Geometry check sheet. Reference: the model listing, model coordinates, mm. A direction names the side the tool comes from. Round coordinates to 2 decimals unless told otherwise and drop trailing zeros. Loops run counter-clockwise (first coordinate to the right, second up) from the corner with the lowest first, then second, coordinate; pieces in that order, holes last. Notation, with made-up numbers: (72.25, 40.5) - (112.25, 40.5) arc R15 cw to (112.25, 62.5) - close; hole circle Ø9 at (75.5, 75.5). An arc over 180 degrees is marked (long way). Write item = value, one per line.
```python
from build123d import *

# Parameters (mm, degrees)
EXTRUDE_1_DEPTH = 1.5
EXTRUDE_2_DEPTH = 1
FILLET_1_R      = 0.5


with BuildPart() as part:
    # 草图1 → 凸台-拉伸1 (new body)
    with BuildSketch(Plane(origin=(0, 0, 0), x_dir=(1, 0, 0), z_dir=(0, 1, 0))):
        Polygon((-24.5, 13), (24.5, 13), (24.5, -13), (7.05, -13), (7.05, -26), (7.05, -27.5), (-7.05, -27.5), (-7.05, -26), (-7.05, -13), (-24.5, -13), align=None)
    extrude(amount=EXTRUDE_1_DEPTH)

    # 草图2 → 凸台-拉伸2 (add)
    with BuildSketch(Plane(origin=(0, 1.5, 0), x_dir=(1, 0, 0), z_dir=(0, 1, 0))):
        Polygon((23, 11.5), (23, -11.5), (5.55, -11.5), (5.55, -13), (5.55, -24.5), (5.55, -26), (-5.55, -26), (-5.55, -24.5), (-5.55, -13), (-5.55, -11.5), (-23, -11.5), (-23, 11.5), align=None)
    extrude(amount=EXTRUDE_2_DEPTH)

    # 圆角1
    fillet_1_edges = [part.edges().sort_by_distance(p)[0] for p in [
        (7.05, 0, 20.25),
        (0, 0, 27.5),
        (-7.05, 0, 20.25),
        (-15.775, 0, 13),
        (-24.5, 0, 0),
        (0, 0, -13),
        (24.5, 0, 0),
        (15.775, 0, 13),
    ]]
    fillet(fillet_1_edges, radius=FILLET_1_R)


solid = part.part
```
(1) Gauge pin test, flat ends, axial feed: pin 1 (0.5 mm diameter, centred on y = 1, z = 22.5, fed in from +X); pin 2 (0.5 mm diameter, centred on y = 2, z = -1, fed in from -X); pin 3 (0.8 mm diameter, centred on x = -4.5, y = 2, fed in from -Z). Record the tip position at first contact, or that the pin passes through.
Answers follow:
pin_1 = 7.05
pin_2 = -23
pin_3 = -11.5
(2) Section check C-C (z = 24). Enter the section's corners in (x, y), then the cut area to 3 significant figures.
Answers follow:
outline = (-7.05, 0.5) arc R0.5 ccw to (-6.55, 0) - (6.55, 0) arc R0.5 ccw to (7.05, 0.5) - (7.05, 1.5) - (5.55, 1.5) - (5.55, 2.5) - (-5.55, 2.5) - (-5.55, 1.5) - (-7.05, 1.5) - close
area = 32.1 mm²
(3) Set-up check for faces 1 (the flat face through (16, 1, 13)), 2 (the flat face through (-14, 2, 11.5)), 3 (the flat face through (-23, 2, 0)), 4 (the flat face through (23, 2, 0)): record each of +Z, -Z, +X, -X, +Y, -Y from which the full face is reachable in a straight line by a thin tool's end or side.
Answers follow:
face_1 = +Z, +X, +Y, -Y
face_2 = +Z, -X, +Y
face_3 = +Z, -Z, -X, +Y
face_4 = +Z, -Z, +X, +Y
(4) Section check A-A (y = 1.9). Enter the section's corners in (x, z).
Answers follow:
outline = (-23, -11.5) - (23, -11.5) - (23, 11.5) - (5.55, 11.5) - (5.55, 26) - (-5.55, 26) - (-5.55, 11.5) - (-23, 11.5) - close
(5) Section check B-B (x = 8). Enter the section's corners in (y, z).
Answers follow:
outline = (0, -12.5) arc R0.5 ccw to (0.5, -13) - (1.5, -13) - (1.5, -11.5) - (2.5, -11.5) - (2.5, 11.5) - (1.5, 11.5) - (1.5, 13) - (0.5, 13) arc R0.5 ccw to (0, 12.5) - close
(6) Scan lines: L1, parallel to X at y = 2.15, z = 16.5; L2, parallel to Z at x = -18, y = 2; L3, parallel to Z at x = -9, y = 1.3. Record each from-to range of solid material in increasing order. Write a range as [from, to].
Answers follow:
L1 = [-5.55, 5.55]
L2 = [-11.5, 11.5]
L3 = [-13, 13]
